```python
from build123d import *

# Parameters (mm, degrees)
F0_W     = 17.5
F0_H     = 2
F0_W_2   = 18.5
F0_W_3   = 4.5
F0_W_4   = 2
F0_H_2   = 25
F0_W_5   = 21
F1_DEPTH = 2
F2_DEPTH = 14.5
F3_DEPTH = 11.5
F4_DEPTH = 8.5
F5_DEPTH = 5


with BuildPart() as f1:
    # F0 (on Front) → F1 (new body)
    with BuildSketch(Plane.XZ):
        with Locations((11.5, 31)):
            Rectangle(F0_W, F0_H)
        with Locations((2.5, -31)):
            Rectangle(F0_W_2, F0_H)
        Polygon((43, 18.75), (43, 32), (20.25, 32), (20.25, 30), (41, 30), (41, 18.75), align=None)
        with Locations((0.5, 31)):
            Rectangle(F0_W_3, F0_H)
        with Locations((42, 6.25)):
            Rectangle(F0_W_4, F0_H_2)
        Polygon((43, -32), (43, -6.25), (41, -6.25), (41, -30), (11.75, -30), (11.75, -32), align=None)
        with Locations((-12.25, 31)):
            Rectangle(F0_W_5, F0_H)
        Polygon((-22.75, 30), (-22.75, 32), (-43, 32), (-43, -32), (-6.75, -32), (-6.75, -30), (-41, -30), (-41, 30), align=None)
        Polygon((41, 30), (20.25, 30), (2.75, 30), (-1.75, 30), (-22.75, 30), (-41, 30), (-41, -30), (-6.75, -30), (11.75, -30), (41, -30), (41, -6.25), (41, 18.75), align=None)
    extrude(amount=F1_DEPTH)

    # F0 (on Front) → F2 (join)
    with BuildSketch(Plane.XZ):
        with Locations((2.5, -31)):
            Rectangle(F0_W_2, F0_H)
    extrude(amount=-F2_DEPTH)

    # F0 (on Front) → F3 (join)
    with BuildSketch(Plane.XZ):
        with Locations((42, 6.25)):
            Rectangle(F0_W_4, F0_H_2)
    extrude(amount=-F3_DEPTH)

    # F0 (on Front) → F4 (join)
    with BuildSketch(Plane.XZ):
        with Locations((11.5, 31)):
            Rectangle(F0_W, F0_H)
    extrude(amount=-F4_DEPTH)

    # F0 (on Front) → F5 (join)
    with BuildSketch(Plane.XZ):
        with Locations((-12.25, 31)):
            Rectangle(F0_W_5, F0_H)
    extrude(amount=-F5_DEPTH)


solid = f1.part
```
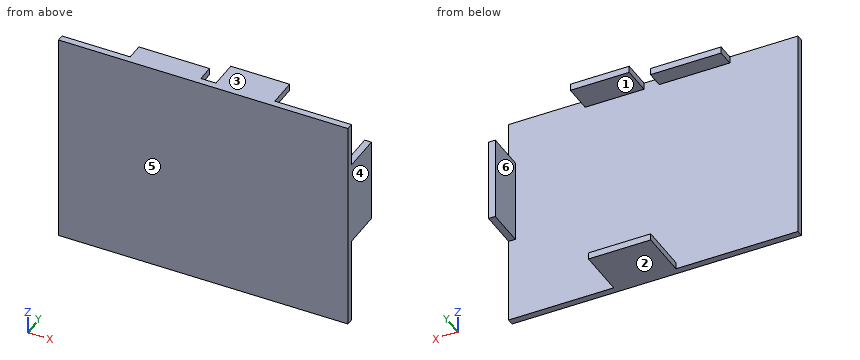
Could you check a few things on this model? Use its own coordinates, in mm. Face numbers are marked on the shaded views. A direction names the side the tool comes from. Give positions to 0.01 mm unless a question says otherwise; leave off trailing zeros. Order: outer loops, then holes, each group sorted by start corner. A loop starts at its lowest first (then second) coordinate and runs counter-clockwise, first axis right, second up.
Q1. Suppose I cut it at D-D, the plane y = 13.5. Write out the boundary of the cut face in (x, z), and give its area (3 significant figures).
Q2. For the marked faces 5 and 6, which set-ups out of +Z, -Z, +X, -X, +Y, -Y let a thin tool reach every point of the face, with its end or its side?
Q3. We'd pull the mould along Z, two halves only. Please class the marked faces 1, 2, 3 and 4: +Z half, -Z half, draft (parallel to the pull), parting line (faces both ways), or undercut.
Q4. I'm going to push flat-ended pins straight in: P1, Ø1.5, axis at x = -8.5, y = 3.5, coming from the -Z side; P2, Ø10, axis at x = -8, z = 22.5, coming from the +Y side; P3, Ø1, axis at y = 3.5, z = 31, coming from the -X side. Where does each tip first touch, or does it pass through?
Q5. Suppose I cut it at B-B, the plane x = -17.5. Write out the boundary of the cut face in (y, z), and give its area (3 significant figures).
Q6. Suppose I cut it at A-A, the plane y = 6.25. Write out the boundary of the cut face in (x, z), and give its area (3 significant figures).
Q7. If I drill on line 1 along Z through (x, y) = (-3, 3.75); line 2 along Y through (x, z) = (24.5, -12); line 3 along Z through (x, y) = (1.5, 6.5), over which ranges is the centre line in solid material (lowest first)?
Q8. Suppose I cut it at C-C, the plane z = 12. Write out the boundary of the cut face in (x, y).
Solution:
1. outline: (-6.75, -32) - (11.75, -32) - (11.75, -30) - (-6.75, -30) - close
1. area: 37.0 mm2
2. face 5: +Z, -Z, +X, -X, -Y
2. face 6: +Z, -Z, -X, +Y
3. face 1: undercut
3. face 2: -Z half
3. face 3: +Z half
3. face 4: draft
4. P1: stops at z = 30
4. P2: stops at y = 0
4. P3: stops at x = -22.75
5. outline: (-2, -32) - (0, -32) - (0, 30) - (5, 30) - (5, 32) - (-2, 32) - close
5. area: 138 mm2
6. outline: (-6.75, -32) - (11.75, -32) - (11.75, -30) - (-6.75, -30) - close; (2.75, 30) - (20.25, 30) - (20.25, 32) - (2.75, 32) - close; (41, -6.25) - (43, -6.25) - (43, 18.75) - (41, 18.75) - close
6. area: 122 mm2
7. line 1: z = -32 to -30, 30 to 32
7. line 2: y = -2 to 0
7. line 3: z = -32 to -30
8. outline: (-43, -2) - (43, -2) - (43, 11.5) - (41, 11.5) - (41, 0) - (-43, 0) - close
